Check sheet for the drawn part. Datum: minimum x, y, z corner. Units: mm. Round coordinates to 2 decimals unless told otherwise and drop trailing zeros. Loops run counter-clockwise (first coordinate to the right, second up) from the corner with the lowest first, then second, coordinate; pieces in that order, holes last.
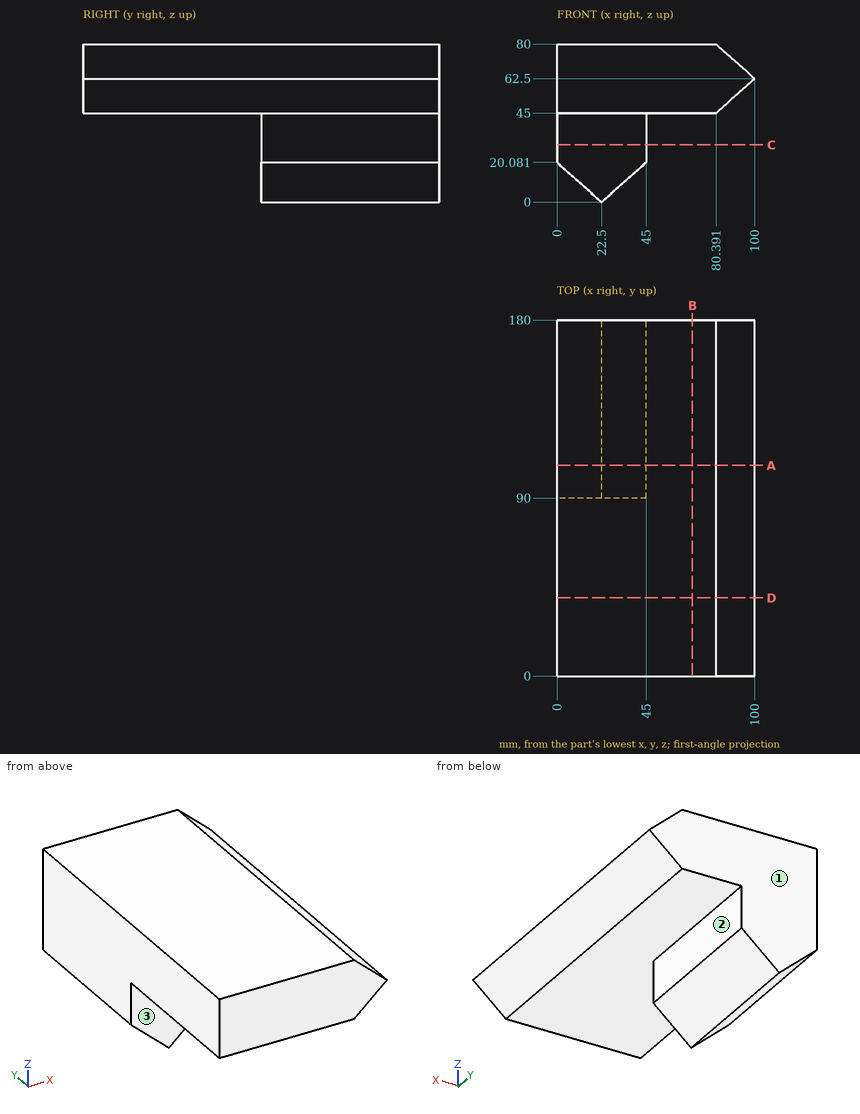
1) Sectioned sample at B-B, the plane x = 68.5. Record the cut outline in (y, z), then the cut area to 3 significant figures.
Report:
outline: (0, 45) - (180, 45) - (180, 80) - (0, 80) - close
area: 6,300 mm2
2) Scan lines: line 1 along X through (y, z) = (148.5, 28.5); line 2 along Y through (x, z) = (26.5, 27); line 3 along Z through (x, y) = (69, 140.5). Record each from-to range of solid material in increasing order.
Report:
line 1: x = 0 to 45
line 2: y = 90 to 180
line 3: z = 45 to 80
3) Mould release check, pull along Y, two halves, no side actions. Record for the marked faces 1, 2 and 3: +Y half, -Y half, draft (parallel to the pull), parting line (faces both ways), or undercut.
Report:
face 1: +Y half
face 2: draft
face 3: -Y half
4) Sectioned sample at C-C, the plane z = 29. Record the cut outline in (x, y).
Report:
outline: (0, 90) - (45, 90) - (45, 180) - (0, 180) - close
5) Sectioned sample at D-D, the plane y = 39.5. Record the cut outline in (x, z), then the cut area to 3 significant figures.
Report:
outline: (0, 45) - (80.39, 45) - (100, 62.5) - (80.39, 80) - (0, 80) - close
area: 3,160 mm2
6) Gauge pin test, flat ends, axial feed: pin 1 (12.5 mm diameter, centred on y = 145.5, z = 31, fed in from +X); pin 2 (5 mm diameter, centred on x = 89.5, y = 35.5, fed in from +Z); pin 3 (3 mm diameter, centred on x = 86.5, y = 98.5, fed in from +Z). Record the tip position at first contact, or that the pin passes through.
Report:
pin 1: stops at x = 45
pin 2: stops at z = 74.1
pin 3: stops at z = 75.89
7) Sectioned sample at A-A, the plane y = 106.5. Record the cut outline in (x, z).
Report:
outline: (0, 20.08) - (22.5, 0) - (45, 20.08) - (45, 45) - (80.39, 45) - (100, 62.5) - (80.39, 80) - (0, 80) - close
